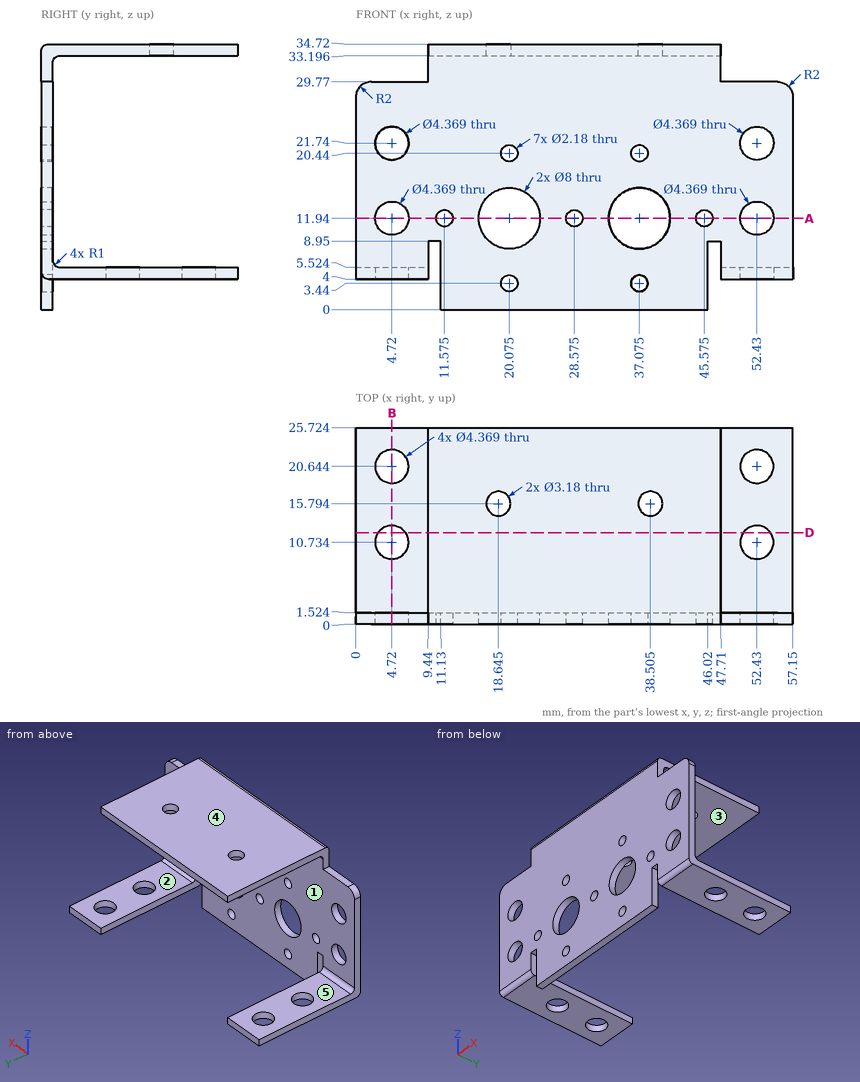
Here's the drawing with two shaded views (mm, measured from the low corner). I have some questions. A direction names the side the tool comes from. Round coordinates to 2 decimals unless told otherwise and drop trailing zeros. Write each loop counter-clockwise with the first axis right and the second up, starting at its lowest first coordinate (ties: lowest second). Pieces come first, ordered by that corner, then holes.
(1) Suppose I cut it at D-D on y = 12. Write out the boundary of the cut face in (x, z).
Findings below:
outline: (0, 4) - (2.94, 4) - (2.94, 5.52) - (0, 5.52) - close; (6.5, 4) - (9.44, 4) - (9.44, 5.52) - (6.5, 5.52) - close; (9.44, 33.2) - (47.71, 33.2) - (47.71, 34.72) - (9.44, 34.72) - close; (47.71, 4) - (50.65, 4) - (50.65, 5.52) - (47.71, 5.52) - close; (54.21, 4) - (57.15, 4) - (57.15, 5.52) - (54.21, 5.52) - close
(2) For pin 1 (1.5 mm diameter, centred on x = 18, y = 5, fed in from -Z); pin 2 (3 mm diameter, centred on x = 4.5, y = 10, fed in from +Z); pin 3 (0.8 mm diameter, centred on y = 0.5, z = 3.5, fed in from -X); pin 4 (4 mm diameter, centred on x = 52.43, y = 10.734, fed in from -Z), each with a flat end and sliding along its axis, tell me the tip position at first contact or that it passes through.
Findings below:
pin 1: stops at z = 33.2
pin 2: stops at z = 5.52
pin 3: stops at x = 11.13
pin 4: passes through
(3) Thinking about a two-plate mould opening in Z: for the marked faces 1, 2 and 3, which applies, +Z half, -Z half, draft (parallel to the pull), parting line (faces both ways), or undercut?
Findings below:
face 1: draft
face 2: +Z half
face 3: -Z half
(4) Which directions (+Z, -Z, +X, -X, +Y, -Y) give clear straight access to the entire face, cutting with the end or side of a thin tool? Please do the marked faces 4 and 5.
Findings below:
face 4: +Z, +X, -X, +Y, -Y
face 5: +Z, +X, -X, +Y
(5) Suppose I cut it at B-B on x = 4.72. Write out the boundary of the cut face in (y, z).
Findings below:
outline: (0, 5) arc R1 ccw to (1, 4) - (8.55, 4) - (8.55, 5.52) - (2.52, 5.52) arc R1 cw to (1.52, 6.52) - (1.52, 9.76) - (0, 9.76) - close; (0, 14.12) - (1.52, 14.12) - (1.52, 19.56) - (0, 19.56) - close; (0, 23.92) - (1.52, 23.92) - (1.52, 29.77) - (0, 29.77) - close; (12.92, 4) - (18.46, 4) - (18.46, 5.52) - (12.92, 5.52) - close; (22.83, 4) - (25.72, 4) - (25.72, 5.52) - (22.83, 5.52) - close
(6) Suppose I cut it at A-A on z = 11.94. State how many separate pieces and enclosed holes the cut face has.
Findings below:
separate pieces: 8
enclosed holes: 0
(7) If I drill on probe 1 along X at (y, z) = (0.7, 21.74); probe 2 along Z at (x, y) = (52.43, 0.3) (1 decimal); probe 3 along X at (y, z) = (0.7, 3.44) (3 decimals), over which ranges is the centre line in solid material (lowest first)?
Findings below:
probe 1: x = 0 to 2.54, 6.9 to 50.25, 54.61 to 57.15
probe 2: z = 4.3 to 9.8, 14.1 to 19.6, 23.9 to 29.8
probe 3: x = 11.13 to 18.985, 21.165 to 35.985, 38.165 to 46.02
